Source: CAD feature listing. Evaluate the final solid. Frame: model axes, mm. Coordinates: 2 decimals unless noted, no trailing zeros. Loops run counter-clockwise (first coordinate to the right, second up) from the corner with the lowest first, then second, coordinate; pieces in that order, holes last. Notation, with made-up numbers: (-24.5, 14.5) -> (16.5, 14.5) arc R20 ccw to (16.5, 48.5) -> close; hole circle Ø8 at (34.25, 52). An arc over 180 degrees is marked (long way). Answer as CSV lines item,"result".
from build123d import *

# Parameters (mm, degrees)
ESQUISSE1_W        = 128.5
ESQUISSE1_H        = 50.5
ESQUISSE1_R        = 1.6
ESQUISSE1_R_2      = 5
BOSS_EXTRU_1_DEPTH = 1


with BuildPart() as part:
    # Esquisse1 → Boss.-Extru.1 (new body)
    with BuildSketch(Plane.XY):
        Rectangle(ESQUISSE1_W, ESQUISSE1_H)
        with Locations((25, 12.5)):
            Circle(ESQUISSE1_R, mode=Mode.SUBTRACT)
        with Locations((-25, 12.5)):
            Circle(ESQUISSE1_R, mode=Mode.SUBTRACT)
        with Locations((-25, -12.5)):
            Circle(ESQUISSE1_R, mode=Mode.SUBTRACT)
        with Locations((25, -12.5)):
            Circle(ESQUISSE1_R, mode=Mode.SUBTRACT)
        with Locations((12.5, -12.5)):
            Circle(ESQUISSE1_R_2, mode=Mode.SUBTRACT)
        with Locations((-37.5, -12.5)):
            Circle(ESQUISSE1_R_2, mode=Mode.SUBTRACT)
        with Locations((-12.5, -12.5)):
            Circle(ESQUISSE1_R_2, mode=Mode.SUBTRACT)
        with Locations((37.5, -12.5)):
            Circle(ESQUISSE1_R_2, mode=Mode.SUBTRACT)
        with Locations((37.5, 12.5)):
            Circle(ESQUISSE1_R_2, mode=Mode.SUBTRACT)
        with Locations((12.5, 12.5)):
            Circle(ESQUISSE1_R_2, mode=Mode.SUBTRACT)
        with Locations((-12.5, 12.5)):
            Circle(ESQUISSE1_R_2, mode=Mode.SUBTRACT)
        with Locations((-37.5, 12.5)):
            Circle(ESQUISSE1_R_2, mode=Mode.SUBTRACT)
        with BuildLine():
            ThreePointArc((62.85, -17.25), (61.25, -15.65), (59.65, -17.25))
            Line((59.65, -17.25), (59.65, -18.25))
            ThreePointArc((59.65, -18.25), (61.25, -19.85), (62.85, -18.25))
            Line((62.85, -18.25), (62.85, -17.25))
        make_face(mode=Mode.SUBTRACT)
        with BuildLine():
            ThreePointArc((59.65, 17.25), (61.25, 15.65), (62.85, 17.25))
            Line((62.85, 17.25), (62.85, 18.25))
            ThreePointArc((62.85, 18.25), (61.25, 19.85), (59.65, 18.25))
            Line((59.65, 18.25), (59.65, 17.25))
        make_face(mode=Mode.SUBTRACT)
        with BuildLine():
            ThreePointArc((-59.65, -17.25), (-61.25, -15.65), (-62.85, -17.25))
            Line((-62.85, -17.25), (-62.85, -18.25))
            ThreePointArc((-62.85, -18.25), (-61.25, -19.85), (-59.65, -18.25))
            Line((-59.65, -18.25), (-59.65, -17.25))
        make_face(mode=Mode.SUBTRACT)
        with BuildLine():
            ThreePointArc((-59.65, 18.25), (-61.25, 19.85), (-62.85, 18.25))
            Line((-62.85, 18.25), (-62.85, 17.25))
            ThreePointArc((-62.85, 17.25), (-61.25, 15.65), (-59.65, 17.25))
            Line((-59.65, 17.25), (-59.65, 18.25))
        make_face(mode=Mode.SUBTRACT)
    extrude(amount=BOSS_EXTRU_1_DEPTH)


solid = part.part
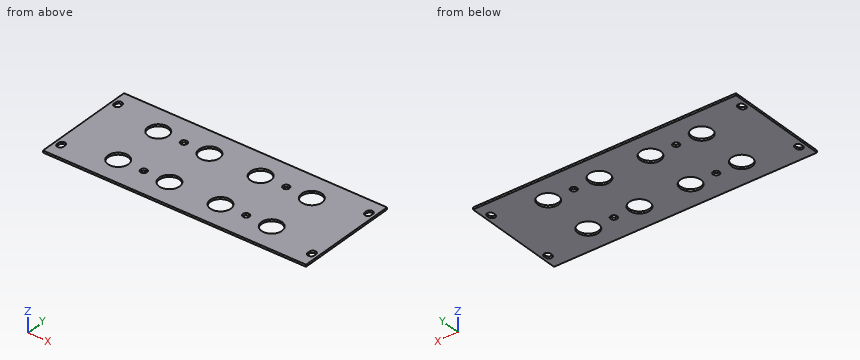
(1) Cut plane B-B (y = -9.5). Return the cut outline in (x, z).
Computed values:
outline,"(-64.25, 0) -> (-41.5, 0) -> (-41.5, 1) -> (-64.25, 1) -> close; (-33.5, 0) -> (-16.5, 0) -> (-16.5, 1) -> (-33.5, 1) -> close; (-8.5, 0) -> (8.5, 0) -> (8.5, 1) -> (-8.5, 1) -> close; (16.5, 0) -> (33.5, 0) -> (33.5, 1) -> (16.5, 1) -> close; (41.5, 0) -> (64.25, 0) -> (64.25, 1) -> (41.5, 1) -> close"
(2) Cut plane D-D (x = 25). Return the cut outline in (y, z).
Computed values:
outline,"(-25.25, 0) -> (-14.1, 0) -> (-14.1, 1) -> (-25.25, 1) -> close; (-10.9, 0) -> (10.9, 0) -> (10.9, 1) -> (-10.9, 1) -> close; (14.1, 0) -> (25.25, 0) -> (25.25, 1) -> (14.1, 1) -> close"
(3) Material intervals for L1, parallel to X at y = -18, z = 0.5; L2, parallel to Y at x = -25, z = 0.3; L3, parallel to Y at x = -12.5, z = 0.3, sorted ascending. Write a range as [from, to].
Computed values:
L1,"[-64.25, -62.85], [-59.65, 59.65], [62.85, 64.25]"
L2,"[-25.25, -14.1], [-10.9, 10.9], [14.1, 25.25]"
L3,"[-25.25, -17.5], [-7.5, 7.5], [17.5, 25.25]"
(4) Cut plane A-A (x = 61.25). Return the cut outline in (y, z), then the cut area to 3 significant figures.
Computed values:
outline,"(-25.25, 0) -> (-19.85, 0) -> (-19.85, 1) -> (-25.25, 1) -> close; (-15.65, 0) -> (15.65, 0) -> (15.65, 1) -> (-15.65, 1) -> close; (19.85, 0) -> (25.25, 0) -> (25.25, 1) -> (19.85, 1) -> close"
area,"42.1 mm^2"
(5) Cut plane C-C (z = 0.5). State how many separate pieces and enclosed holes the cut face has, then the cut area to 3 significant figures.
Computed values:
separate pieces,"1"
enclosed holes,"16"
area,"5,780 mm^2"
